The model under review builds one solid part; all positions refer to its coordinate system, in mm. A direction names the side the tool comes from. Give positions to 0.01 mm unless a question says otherwise; leave off trailing zeros. Order: outer loops, then holes, each group sorted by start corner. A loop starts at its lowest first (then second) coordinate and runs counter-clockwise, first axis right, second up. Notation, with made-up numbers: M 0.5,-38.75 L 43.5,-38.75 A13 cw 43.5,-28.75 Z; hole C 31.25,16 d1. An arc over 180 degrees is marked long. One line per question, with ' | ' between items. Start each with the question number.
1. We need section B-B on y = 105. Write out the cut boundary in (x, z) (3 decimals).
2. The part is to be moulded in two halves that separate along X. For faces 4 (the face through (-14, 8, 131)), 5 (the face through (-24.471, 99, 132)), 6 (the face through (39.779, 84, 83)), 7 (the face through (60, 67, -15.875)), say which applies: +X half, -X half, draft (parallel to the pull), parting line (faces both ways), or undercut.
3. Wall thickness on L1, parallel to Z at x = -14, y = 49.5 (3 decimals); L2, parallel to Z at x = -16, y = 40 (3 decimals); L3, parallel to X at y = 105, z = 138.35: over which ranges is each line inside the solid? List them lowest first.
4. We need section C-C on z = 92.5. Write out the cut boundary in (x, y), then the cut area to 3 significant figures.
5. Insertion check: P1, Ø2, axis at x = 15, y = 52, coming from the +Z side (3 decimals); P2, Ø6, axis at x = 14, z = 80.5, coming from the +Y side; P3, Ø2.5, axis at y = 85.5, z = 83, coming from the -X side. Each pin has a flat end and moves straight along its axis. Give the tip position at first contact, or say it passes through.
6. We need section A-A on x = 50. Write out the cut boundary in (y, z) (3 decimals).
7. For faces 1 (the face through (-14, 99, 141.975)), 2 (the face through (11.925, 19.056, 131.251)), 3 (the face through (-14, 64, 138)), list the 3-axis set-ups (+Z, -Z, +X, -X, +Y, -Y) from which the entire face can be reached by the end or side of a thin tool; tool diameter is ignored.
```python
from build123d import *

# Parameters (mm, degrees)
SKETCH1_W                                           = 155.7
SKETCH1_H                                           = 155.7
BOSS_EXTRUDE2_DEPTH                                 = 80
SKETCH3_W                                           = 8
SKETCH3_H                                           = 25
BOSS_EXTRUDE4_DEPTH                                 = 145.45
CHAMFER1_SIZE                                       = 0.508
CHAMFER1_SIZE2                                      = 0.03552282
CHAMFER2_SIZE                                       = 0.508
CHAMFER2_SIZE2                                      = 0.03552282
SKETCH4_W                                           = 8.2
SKETCH4_H                                           = 25.2
CUT_EXTRUDE6_DEPTH                                  = 160.2
FILLET1_R                                           = 1
SKETCH6_W                                           = 10.35
SKETCH6_H                                           = 10.25
CUT_EXTRUDE7_DEPTH                                  = 80
SKETCH7_W                                           = 10.25
SKETCH7_H                                           = 10.25
BOSS_EXTRUDE5_DEPTH                                 = 80
CSK_FOR_M3_COUNTERSUNK_FLAT_HEAD_SCREW1_D           = 3.4
CSK_FOR_M3_COUNTERSUNK_FLAT_HEAD_SCREW1_DEPTH       = 16
CSK_FOR_M3_COUNTERSUNK_FLAT_HEAD_SCREW1_CSINK_D     = 6.3
CSK_FOR_M3_COUNTERSUNK_FLAT_HEAD_SCREW1_CSINK_ANGLE = 90
CSK_FOR_M3_COUNTERSUNK_FLAT_HEAD_SCREW1_TIP         = 1.021463052
SKETCH12_R                                          = 2.1
CUT_EXTRUDE9_DEPTH                                  = 5
FILLET2_START                                       = -18.821212121
FILLET2_DEPTH                                       = 152.821212121
FILLET3_START                                       = -18.821212121
FILLET3_DEPTH                                       = 152.821212121
SKETCH14_W                                          = 9.8
SKETCH14_H                                          = 9.8
BOSS_EXTRUDE6_DEPTH                                 = 8
CUT_EXTRUDE12_START                                 = -9.8
SKETCH17_W                                          = 6
SKETCH17_H                                          = 1
CUT_EXTRUDE12_DEPTH                                 = 1
CUT_EXTRUDE13_START                                 = -9.8
SKETCH19_W                                          = 6
SKETCH19_H                                          = 1
CUT_EXTRUDE13_DEPTH                                 = 1
BOSS_EXTRUDE7_DEPTH                                 = 5
BOSS_EXTRUDE7_DEPTH_BACK                            = 80
SKETCH20_W                                          = 25
SKETCH20_H                                          = 25
SKETCH21_W                                          = 20.8
SKETCH21_H                                          = 20.8
BOSS_EXTRUDE8_DEPTH                                 = 38
SKETCH23_W                                          = 12.85
SKETCH23_H                                          = 12.85
CUT_EXTRUDE14_DEPTH                                 = 110
CSK_FOR_M4_COUNTERSUNK_FLAT_HEAD_SCREW1_D           = 4.5
CSK_FOR_M4_COUNTERSUNK_FLAT_HEAD_SCREW1_DEPTH       = 26
CSK_FOR_M4_COUNTERSUNK_FLAT_HEAD_SCREW1_CSINK_D     = 9.4
CSK_FOR_M4_COUNTERSUNK_FLAT_HEAD_SCREW1_CSINK_ANGLE = 90
CSK_FOR_M4_COUNTERSUNK_FLAT_HEAD_SCREW1_TIP         = 1.351936393
SKETCH27_W                                          = 8
SKETCH27_H                                          = 8
CUT_EXTRUDE15_DEPTH                                 = 20
SKETCH28_W                                          = 10
SKETCH28_H                                          = 8
CUT_EXTRUDE16_DEPTH                                 = 33.925
FILLET4_R                                           = 5
FILLET5_R                                           = 3


with BuildPart() as part:
    # Sketch1 → Boss-Extrude2 (new body)
    with BuildSketch(Plane(origin=(0, 0, 0), x_dir=(1, 0, 0), z_dir=(0, 1, 0))):
        with Locations((55.528787879, -61.975)):
            Rectangle(SKETCH1_W, SKETCH1_H)
    extrude(amount=BOSS_EXTRUDE2_DEPTH)

    # Sketch3 → Boss-Extrude4 (add)
    with BuildSketch(Plane.XY.offset(-15.875)):
        with Locations((137.378787879, 40)):
            Rectangle(SKETCH3_W, SKETCH3_H)
    extrude(amount=BOSS_EXTRUDE4_DEPTH)

    # Chamfer1
    chamfer1_edges = [part.edges().sort_by_distance(p)[0] for p in [
        (141.378787879, 52.5, 56.85),
    ]]
    chamfer1_side = [part.faces().sort_by_distance(p)[0] for p in [
        (137.378787879, 52.5, 56.85),
    ]]
    chamfer(chamfer1_edges, length=CHAMFER1_SIZE, length2=CHAMFER1_SIZE2, reference=chamfer1_side[0])

    # Chamfer2
    chamfer2_edges = [part.edges().sort_by_distance(p)[0] for p in [
        (141.378787879, 27.5, 56.85),
    ]]
    chamfer2_side = [part.faces().sort_by_distance(p)[0] for p in [
        (137.378787879, 27.5, 56.85),
    ]]
    chamfer(chamfer2_edges, length=CHAMFER2_SIZE, length2=CHAMFER2_SIZE2, reference=chamfer2_side[0])

    # Sketch4 → Cut-Extrude6 (cut)
    with BuildSketch(Plane.ZY.offset(-141.378787879)):
        with Locations((-11.775, 40)):
            Rectangle(SKETCH4_W, SKETCH4_H)
    extrude(amount=CUT_EXTRUDE6_DEPTH, mode=Mode.SUBTRACT)

    # Fillet1
    fillet1_edges = [part.edges().sort_by_distance(p)[0] for p in [
        (141.378787879, 40, -7.675),
    ]]
    fillet(fillet1_edges, radius=FILLET1_R)

    # Sketch6 → Cut-Extrude7 (cut)
    with BuildSketch(Plane(origin=(0, 80, 0), x_dir=(1, 0, 0), z_dir=(0, 1, 0))):
        with Locations((128.203787879, -134.7)):
            Rectangle(SKETCH6_W, SKETCH6_H)
    extrude(amount=-CUT_EXTRUDE7_DEPTH, mode=Mode.SUBTRACT)

    # Sketch7 → Boss-Extrude5 (add)
    with BuildSketch(Plane(origin=(0, 80, 0), x_dir=(1, 0, 0), z_dir=(0, 1, 0))):
        with Locations((-17.196212121, 21)):
            Rectangle(SKETCH7_W, SKETCH7_H)
    extrude(amount=-BOSS_EXTRUDE5_DEPTH)

    # CSK for M3 Countersunk Flat Head Screw1
    with Locations(Plane.ZY.offset(22.321212121)):
        with Locations((-21, 40)):
            CounterSinkHole(CSK_FOR_M3_COUNTERSUNK_FLAT_HEAD_SCREW1_D / 2, CSK_FOR_M3_COUNTERSUNK_FLAT_HEAD_SCREW1_CSINK_D / 2, depth=CSK_FOR_M3_COUNTERSUNK_FLAT_HEAD_SCREW1_DEPTH, counter_sink_angle=CSK_FOR_M3_COUNTERSUNK_FLAT_HEAD_SCREW1_CSINK_ANGLE)
            with Locations((0, 0, -(CSK_FOR_M3_COUNTERSUNK_FLAT_HEAD_SCREW1_DEPTH + CSK_FOR_M3_COUNTERSUNK_FLAT_HEAD_SCREW1_TIP / 2))):  # 118° drill point
                Cone(0, CSK_FOR_M3_COUNTERSUNK_FLAT_HEAD_SCREW1_D / 2, CSK_FOR_M3_COUNTERSUNK_FLAT_HEAD_SCREW1_TIP, mode=Mode.SUBTRACT)

    # Sketch12 → Cut-Extrude9 (cut)
    with BuildSketch(Plane.XY.offset(129.575)):
        with Locations((128.203787879, 40)):
            Circle(SKETCH12_R)
    extrude(amount=-CUT_EXTRUDE9_DEPTH, mode=Mode.SUBTRACT)

    # Fillet2: read off the stored shape, not the designer's step
    # Fillet2 outline → Fillet2 (cut)
    with BuildSketch(Plane.YZ.offset(FILLET2_START)):
        with BuildLine():
            Line((52.6, -15.875), (53.6, -15.875))
            ThreePointArc((53.6, -15.875), (52.892893219, -15.582106781), (52.6, -14.875))
            Line((52.6, -14.875), (52.6, -15.875))
        make_face()
    extrude(amount=FILLET2_DEPTH, mode=Mode.SUBTRACT)

    # Fillet3: read off the stored shape, not the designer's step
    # Fillet3 outline → Fillet3 (cut)
    with BuildSketch(Plane.YZ.offset(FILLET3_START)):
        with BuildLine():
            ThreePointArc((27.4, -14.875), (27.107106781, -15.582106781), (26.4, -15.875))
            Line((26.4, -15.875), (27.4, -15.875))
            Line((27.4, -15.875), (27.4, -14.875))
        make_face()
    extrude(amount=FILLET3_DEPTH, mode=Mode.SUBTRACT)

    # Sketch14 → Boss-Extrude6 (add)
    with BuildSketch(Plane(origin=(0, 80, 0), x_dir=(1, 0, 0), z_dir=(0, 1, 0))):
        with Locations((34.878787879, -82.625)):
            Rectangle(SKETCH14_W, SKETCH14_H)
    extrude(amount=BOSS_EXTRUDE6_DEPTH)

    # Sketch17 → Cut-Extrude12 (cut)
    with BuildSketch(Plane(origin=(39.778787879, 0, 0), x_dir=(0, 0, -1), z_dir=(1, 0, 0)).offset(CUT_EXTRUDE12_START)):
        with Locations((-82.625, 85.5)):
            Rectangle(SKETCH17_W, SKETCH17_H)
    extrude(amount=CUT_EXTRUDE12_DEPTH, mode=Mode.SUBTRACT)

    # Sketch19 → Cut-Extrude13 (cut)
    with BuildSketch(Plane(origin=(0, 0, 77.725), x_dir=(-1, 0, 0), z_dir=(0, 0, -1)).offset(CUT_EXTRUDE13_START)):
        with Locations((-34.878787879, 85.5)):
            Rectangle(SKETCH19_W, SKETCH19_H)
    extrude(amount=CUT_EXTRUDE13_DEPTH, mode=Mode.SUBTRACT)

    # Sketch20 → Boss-Extrude7 (add, two sides: drawn at the far end of the back side and taken through both)
    with BuildSketch(Plane(origin=(0, 0, 0), x_dir=(-1, 0, 0), z_dir=(0, -1, 0)).offset(-BOSS_EXTRUDE7_DEPTH_BACK)):
        with Locations((14.071212121, -131.575)):
            Rectangle(SKETCH20_W, SKETCH20_H)
    extrude(amount=BOSS_EXTRUDE7_DEPTH + BOSS_EXTRUDE7_DEPTH_BACK)

    # Sketch21 → Boss-Extrude8 (add)
    with BuildSketch(Plane(origin=(0, 80, 0), x_dir=(1, 0, 0), z_dir=(0, 1, 0))):
        with Locations((-14.071212121, -131.575)):
            Rectangle(SKETCH21_W, SKETCH21_H)
    extrude(amount=BOSS_EXTRUDE8_DEPTH)

    # Sketch23 → Cut-Extrude14 (cut)
    with BuildSketch(Plane(origin=(0, 118, 0), x_dir=(1, 0, 0), z_dir=(0, 1, 0))):
        with Locations((-14.071212121, -131.575)):
            Rectangle(SKETCH23_W, SKETCH23_H)
    extrude(amount=-CUT_EXTRUDE14_DEPTH, mode=Mode.SUBTRACT)

    # CSK for M4 Countersunk Flat Head Screw1
    with Locations(Plane.XY.offset(141.975)):
        with Locations((-14.071212121, 105)):
            CounterSinkHole(CSK_FOR_M4_COUNTERSUNK_FLAT_HEAD_SCREW1_D / 2, CSK_FOR_M4_COUNTERSUNK_FLAT_HEAD_SCREW1_CSINK_D / 2, depth=CSK_FOR_M4_COUNTERSUNK_FLAT_HEAD_SCREW1_DEPTH, counter_sink_angle=CSK_FOR_M4_COUNTERSUNK_FLAT_HEAD_SCREW1_CSINK_ANGLE)
            with Locations((0, 0, -(CSK_FOR_M4_COUNTERSUNK_FLAT_HEAD_SCREW1_DEPTH + CSK_FOR_M4_COUNTERSUNK_FLAT_HEAD_SCREW1_TIP / 2))):  # 118° drill point
                Cone(0, CSK_FOR_M4_COUNTERSUNK_FLAT_HEAD_SCREW1_D / 2, CSK_FOR_M4_COUNTERSUNK_FLAT_HEAD_SCREW1_TIP, mode=Mode.SUBTRACT)

    # Sketch27 → Cut-Extrude15 (cut)
    with BuildSketch(Plane.XY.offset(139.825)):
        with Locations((17.428787879, 19)):
            Rectangle(SKETCH27_W, SKETCH27_H)
    extrude(amount=-CUT_EXTRUDE15_DEPTH, mode=Mode.SUBTRACT)

    # Sketch28 → Cut-Extrude16 (cut)
    with BuildSketch(Plane(origin=(13.428787879, 0, 0), x_dir=(0, 0, -1), z_dir=(1, 0, 0))):
        with Locations((-124.825, 19)):
            Rectangle(SKETCH28_W, SKETCH28_H)
    extrude(amount=-CUT_EXTRUDE16_DEPTH, mode=Mode.SUBTRACT)

    # Fillet4
    fillet4_edges = [part.edges().sort_by_distance(p)[0] for p in [
        (13.428787879, 19, 129.825),
    ]]
    fillet(fillet4_edges, radius=FILLET4_R)

    # Fillet5
    fillet5_edges = [part.edges().sort_by_distance(p)[0] for p in [
        (-7.646212121, 19, 129.825),
    ]]
    fillet(fillet5_edges, radius=FILLET5_R)


solid = part.part
```
Entries:
1) outline: M -24.471,121.175 L -16.321,121.175 L -16.321,125.15 L -20.496,125.15 L -20.496,138 L -16.321,138 L -16.321,139.525 L -18.771,141.975 L -24.471,141.975 Z; M -11.821,121.175 L -3.671,121.175 L -3.671,141.975 L -9.371,141.975 L -11.821,139.525 L -11.821,138 L -7.646,138 L -7.646,125.15 L -11.821,125.15 Z
2) face 4: undercut | face 5: -X half | face 6: +X half | face 7: draft
3) L1: z = -26.125 to -15.875, -7.675 to 125.15, 138 to 144.075 | L2: z = -26.125 to -22.7, -19.3 to -15.875, -7.675 to 125.15, 138 to 144.075 | L3: x = -24.47 to -16.32, -11.82 to -3.67
4) outline: M -22.32,0 L 133.38,0 L 133.38,27.5 L 140.87,27.5 L 141.38,27.54 L 141.38,52.46 L 140.87,52.5 L 133.38,52.5 L 133.38,80 L -22.32,80 Z | area: 12,700 mm^2
5) P1: stops at z = 139.825 | P2: stops at y = 80 | P3: stops at x = 29.98
6) outline: M 0,-15.875 L 26.4,-15.875 A1 ccw 27.4,-14.875 L 27.4,-7.675 L 52.6,-7.675 L 52.6,-14.875 A1 ccw 53.6,-15.875 L 80,-15.875 L 80,139.825 L 0,139.825 Z
7) face 1: +Z, +X, -X, +Y | face 2: none | face 3: +Y
